Verification items for the finished model (mm, model axes). Coordinates: 2 decimals unless noted, no trailing zeros. Write each loop counter-clockwise with the first axis right and the second up, starting at its lowest first coordinate (ties: lowest second). Pieces come first, ordered by that corner, then holes. Notation, with made-up numbers: (58, 72.25) -> (91, 72.25) arc R35 ccw to (91, 107.25) -> close; hole circle Ø10 at (65.5, -2). An arc over 180 degrees is marked (long way). Answer in a Markdown table with one row per item.
Autodesk Inventor part; units mm, degrees
ref_plane "YZ Plane" through (0, 0, 0) normal (1, 0, 0) x (0, 1, 0)
ref_plane "XZ Plane" through (0, 0, 0) normal (0, 1, 0) x (-1, 0, 0)
ref_plane "XY Plane" through (0, 0, 0) normal (0, 0, 1) x (1, 0, 0)
sketch "Skizze1" plane through (0, 0, 0) normal (0, 0, 1) x (1, 0, 0)
  line L0 (0, -1.9) -> (0, 11.4) construction
  line L1 (-7.5, 0) -> (7.5, 0)
  line L2 (7.5, 0) -> (7.5, 9.5)
  line L3 (7.5, 9.5) -> (-7.5, 9.5)
  line L4 (-7.5, 9.5) -> (-7.5, 0)
  circle A0 centre (-7.5, 6.5) radius 1.5
  line L5 (-12.6, 0) -> (12.6, 0)
  line L6 (-4.5, 6.5) -> (-7.5, 6.5) construction
  line L7 (-4.5, 7) -> (-7.5, 7)
  line L8 (-7.5, 6) -> (-4.5, 6)
  arc A1 (-4.5, 6) -> (-4.5, 7) centre (-4.5, 6.5) ccw
  arc A2 (-7.5, 7) -> (-7.5, 6) centre (-7.5, 6.5) ccw
  circle A3 centre (-4.5, 6.5) radius 1
  circle A4 centre (7.5, 6.5) radius 1.5
  line L9 (4.5, 7) -> (7.5, 7)
  line L10 (7.5, 6) -> (4.5, 6)
  arc A5 (4.5, 7) -> (4.5, 6) centre (4.5, 6.5) ccw
  circle A6 centre (4.5, 6.5) radius 1
  point P0 (0, 0)
  point P1 (0, 0)
  point P2 (-7.5, 8)
  point P3 (-7.5, 5)
  point P4 (-6, 6.5)
  point P5 (6, 6.5)
  point P6 (-6.0858, 7)
  point P7 (-5.366, 7)
  point P8 (-5.366, 6)
  point P9 (-6.0858, 6)
  point P10 (7.5, 5)
  point P11 (6.0858, 6)
  point P12 (5.366, 6)
  point P13 (5.366, 7)
  point P14 (6.0858, 7)
  point P15 (7.5, 8)
  dimension "d2" = 3
  dimension "d0" = 15
  dimension "d1" = 9.5
  dimension "d3" = 3
  dimension "d6" = 1
  dimension "d7" = 2
extrude "Extrusion1" add sketch "Skizze1" along normal blind 500 contours L4 A0 L8 A3 L7 L3 L2 A4 L9 A6 L10 L1
sketch "Skizze2" plane through (-7.5, 9.5, 500) normal (0, 1, 0) x (1, 0, 0)
  line L0 (-3, 500) -> (18, 500)
  line L1 (7.5, 1200) -> (7.5, -200)
  circle A0 centre (7.5, 470) radius 3
  circle A1 centre (7.5, 470) radius 1.75
  point P0 (7.5, 500)
  dimension "d8" = 6
  dimension "d9" = 3.5
  dimension "d10" = 30
extrude "Extrusion2" cut sketch "Skizze2" against normal blind 6
extrude "Extrusion3" cut sketch "Skizze2" against normal blind 15 contours A1 L1 | L1 A1
chamfer "Fase1" distance 1 angle 45 1 edges at (-3, 9.5, 30)
pattern_linear "Rechteckige Anordnung1" count 12 spacing 40 along (0, 0, 1) of "Extrusion2", "Extrusion3", "Fase1"
equation "\"d4\" = Raillänge"
equation "\"Raillänge\" = 500"
properties part number "MGN15 Linear Rail 500mm"
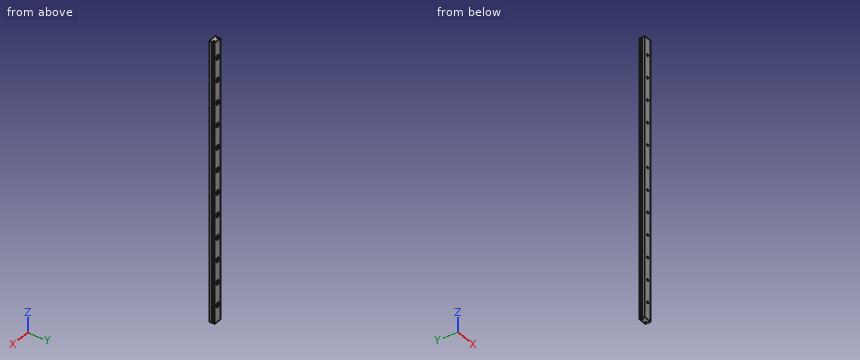
1. Thickness scan on line 1 (Y direction, x = 5.5, z = 44.5); line 2 (Y direction, x = 4.25, z = 50); line 3 (X direction, y = 6.5, z = 70). Record the ranges inside material, lowest first. Write a range as from..to.
Geometry says:
| item | result |
|---|---|
| line 1 | 0..6, 7..9.5 |
| line 2 | 0..5.53, 7.47..9.5 |
| line 3 | -3.5..-3, 3..3.5 |
2. Section check A-A, the plane z = 206. Record the boundary of the cut face in (x, y).
Geometry says:
| item | result |
|---|---|
| outline | (-7.5, 0) -> (7.5, 0) -> (7.5, 5) arc R1.5 cw to (6.09, 6) -> (5.37, 6) arc R1 cw (long way) to (5.37, 7) -> (6.09, 7) arc R1.5 cw to (7.5, 8) -> (7.5, 9.5) -> (-7.5, 9.5) -> (-7.5, 8) arc R1.5 cw to (-6.09, 7) -> (-5.37, 7) arc R1 cw (long way) to (-5.37, 6) -> (-6.09, 6) arc R1.5 cw to (-7.5, 5) -> close |
3. Depth check by flat-ended pin: P1, Ø3, axis at x = 1, z = 390, coming from the +Y side; P2, Ø5, axis at x = -1, z = 230.5, coming from the +Y side; P3, Ø5, axis at x = 0, z = 149, coming from the +Y side. Enter the tip coordinate at first touch or a pass-through.
Geometry says:
| item | result |
|---|---|
| P1 | y = 3.5 |
| P2 | y = 9.12 |
| P3 | y = 9 |
